from build123d import *

# Parameters (mm, degrees)
F0_R     = 1.5
F1_DEPTH = 1.5


# Not quite as in the source:
# - ends of sketch curves that miss each other by under 0.0002 mm in the source are joined


with BuildPart() as f1:
    # F0 (on Top) → F1 (new body)
    with BuildSketch(Plane.XY):
        with BuildLine():
            Line((-29.5, 6.644661), (-29.5, 0))
            Line((-29.5, 0), (-29.5, -6.644661))
            ThreePointArc((-29.5, -6.644661), (-30.4515057083, -11.4282035779), (-33.1611647352, -15.4834952648))
            Line((-33.1611647352, -15.4834952648), (-35.355339, -17.677669))
            Line((-35.355339, -17.677669), (-27.577165, -25.455844))
            ThreePointArc((-27.577165, -25.455844), (-25.4558450782, -25.4558435782), (-25.4558443282, -27.5771636718))
            Line((-25.4558443282, -27.5771636718), (-17.67767, -35.355339))
            ThreePointArc((-17.67767, -35.355339), (-3.536e-07, -28.033008), (17.6776695297, -35.3553384703))
            Line((17.6776695297, -35.3553384703), (25.455844, -27.577164))
            ThreePointArc((25.455844, -27.577164), (25.4558438282, -25.4558438282), (27.5771641718, -25.4558438282))
            Line((27.5771641718, -25.4558438282), (35.355339, -17.677669))
            Line((35.355339, -17.677669), (33.161165, -15.483495))
            ThreePointArc((33.161165, -15.483495), (30.4515057083, -11.4282035779), (29.5, -6.644661))
            Line((29.5, -6.644661), (29.5, 0))
            Line((29.5, 0), (29.5, 6.644661))
            ThreePointArc((29.5, 6.644661), (30.4515058436, 11.4282039046), (33.1611652352, 15.4834957648))
            Line((33.1611652352, 15.4834957648), (35.355339, 17.67767))
            Line((35.355339, 17.67767), (27.577164, 25.455844))
            ThreePointArc((27.577164, 25.455844), (25.4558435782, 25.4558450782), (25.4558438282, 27.5771651718))
            Line((25.4558438282, 27.5771651718), (17.677669, 35.355339))
            ThreePointArc((17.677669, 35.355339), (-3.536e-07, 28.033009), (-17.6776695297, 35.3553394703))
            Line((-17.6776695297, 35.3553394703), (-25.455844, 27.577165))
            ThreePointArc((-25.455844, 27.577165), (-25.4558448282, 25.4558448282), (-27.5771646718, 25.4558443282))
            Line((-27.5771646718, 25.4558443282), (-35.355339, 17.67767))
            Line((-35.355339, 17.67767), (-33.161165, 15.483496))
            ThreePointArc((-33.161165, 15.483496), (-30.4515058436, 11.4282039046), (-29.5, 6.644661))
        make_face()
        with Locations((-17.854446, -26.693281)):
            Circle(F0_R, mode=Mode.SUBTRACT)
        with Locations((-26.693281, -17.854446)):
            Circle(F0_R, mode=Mode.SUBTRACT)
        with Locations((-15.25, -15.25)):
            Circle(F0_R, mode=Mode.SUBTRACT)
        with Locations((17.854446, -26.693281)):
            Circle(F0_R, mode=Mode.SUBTRACT)
        with Locations((26.693281, -17.854446)):
            Circle(F0_R, mode=Mode.SUBTRACT)
        with Locations((15.25, -15.25)):
            Circle(F0_R, mode=Mode.SUBTRACT)
        with BuildLine():
            Line((11.5, -18), (-11.5, -18))
            ThreePointArc((-11.5, -18), (-12.2071067812, -17.7071067812), (-12.5, -17))
            Line((-12.5, -17), (-12.5, -15.25))
            ThreePointArc((-12.5, -15.25), (-13.3054563517, -13.3054563517), (-15.25, -12.5))
            Line((-15.25, -12.5), (-17, -12.5))
            ThreePointArc((-17, -12.5), (-17.7071067812, -12.2071067812), (-18, -11.5))
            Line((-18, -11.5), (-18, 11.5))
            ThreePointArc((-18, 11.5), (-17.7071067812, 12.2071067812), (-17, 12.5))
            Line((-17, 12.5), (-15.25, 12.5))
            ThreePointArc((-15.25, 12.5), (-13.3054563517, 13.3054563517), (-12.5, 15.25))
            Line((-12.5, 15.25), (-12.5, 17))
            ThreePointArc((-12.5, 17), (-12.2071067812, 17.7071067812), (-11.5, 18))
            Line((-11.5, 18), (11.5, 18))
            ThreePointArc((11.5, 18), (12.2071067812, 17.7071067812), (12.5, 17))
            Line((12.5, 17), (12.5, 15.25))
            ThreePointArc((12.5, 15.25), (13.3054563517, 13.3054563517), (15.25, 12.5))
            Line((15.25, 12.5), (17, 12.5))
            ThreePointArc((17, 12.5), (17.7071067812, 12.2071067812), (18, 11.5))
            Line((18, 11.5), (18, -11.5))
            ThreePointArc((18, -11.5), (17.7071067812, -12.2071067812), (17, -12.5))
            Line((17, -12.5), (15.25, -12.5))
            ThreePointArc((15.25, -12.5), (13.3054563517, -13.3054563517), (12.5, -15.25))
            Line((12.5, -15.25), (12.5, -17))
            ThreePointArc((12.5, -17), (12.2071067812, -17.7071067812), (11.5, -18))
        make_face(mode=Mode.SUBTRACT)
        with Locations((-15.25, 15.25)):
            Circle(F0_R, mode=Mode.SUBTRACT)
        with Locations((-26.693281, 17.854447)):
            Circle(F0_R, mode=Mode.SUBTRACT)
        with Locations((-17.854446, 26.693281)):
            Circle(F0_R, mode=Mode.SUBTRACT)
        with Locations((15.25, 15.25)):
            Circle(F0_R, mode=Mode.SUBTRACT)
        with Locations((26.693281, 17.854447)):
            Circle(F0_R, mode=Mode.SUBTRACT)
        with Locations((17.854446, 26.693281)):
            Circle(F0_R, mode=Mode.SUBTRACT)
    extrude(amount=F1_DEPTH)


solid = f1.part
Read the model definition and answer for the solid it produces. Units are mm, in the model's axes. A direction names the side the tool comes from. Give positions to 0.01 mm unless a question says otherwise; leave off trailing zeros. Write each loop counter-clockwise with the first axis right and the second up, starting at its lowest first coordinate (ties: lowest second). Pieces come first, ordered by that corner, then holes. Notation, with made-up numbers: (25.25, 45.25) -> (34.25, 45.25) arc R11 cw to (34.25, 57.25) -> close; hole circle Ø1 at (-3, 89). An arc over 180 degrees is marked (long way). Answer as a JSON object with one key per item and string values. Group by question number.
1) The mould has two halves that part along X. Classify faces 5 (the flat face through (-31.412, 21.621, 0.74)), 6 (the cylindrical face through (-0.275, -28.035, 0.74)), 7 (the cylindrical face through (13.75, -15.18, 0.74)), 8 (the flat face through (34.243, 16.565, 0.74)): +X half, -X half, draft (parallel to the pull), parting line (faces both ways), or undercut.
2) Find section A-A (y = -0.5). Write down the section's boundary in (x, z).
3) Each of these flat-tipped pins is pushed along its axis until it touches: P1, Ø2.5, axis at x = -26.69, y = 17.85, coming from the +Z side; P2, Ø0.8, axis at y = 1, z = 1, coming from the -X side; P3, Ø0.8, axis at y = 1.5, z = 1, coming from the +X side. Where does it stop, or does it pass through?
4) Find section D-D (y = 23). Write down the section's boundary in (x, z).
5) Find section C-C (z = 0.35). Count the separate pieces of the cut face and the enclosed holes in it, and give its area (3 significant figures).
6) A tool of negligible diameter and unlimited length cuts with its end or side. For faces 1 (the cylindrical face through (0.275, 28.035, 0.74)), 2 (the cylindrical face through (13.28, 13.33, 0.74)), 3 (the flat face through (-34.274, 16.596, 0.74)), 4 (the cylindrical face through (30.478, -11.492, 0.74)), from which of +Z, -Z, +X, -X, +Y, -Y can it reach the whole face along a straight path? Write none if from no direction.
7) Find section B-B (x = -2). Write down the section's boundary in (y, z), and give its area (3 significant figures).
8) Consider L1, parallel to Y at x = 26.5, z = 0.5; L2, parallel to X at y = 15.5, z = 1.4; L3, parallel to X at y = 28, z = 0.4. Determine where each line is inside the solid, lowest interval first. Write a range as from..to.
Values follow:
{
 "1": {"face 5": "-X half", "face 6": "undercut", "face 7": "undercut", "face 8": "+X half"},
 "2": {"outline": "(-29.5, 0) -> (-18, 0) -> (-18, 1.5) -> (-29.5, 1.5) -> close; (18, 0) -> (29.5, 0) -> (29.5, 1.5) -> (18, 1.5) -> close"},
 "3": {"P1": "passes through", "P2": "stops at x = -29.5", "P3": "stops at x = 29.5"},
 "4": {"outline": "(-30.03, 0) -> (30.03, 0) -> (30.03, 1.5) -> (-30.03, 1.5) -> close"},
 "5": {"separate pieces": "1", "enclosed holes": "13", "area": "2,410 mm2"},
 "6": {"face 1": "+Z, -Z, +Y", "face 2": "+Z, -Z", "face 3": "+Z, -Z, -X", "face 4": "+Z, -Z, +X"},
 "7": {"outline": "(-28.11, 0) -> (-18, 0) -> (-18, 1.5) -> (-28.11, 1.5) -> close; (18, 0) -> (28.11, 0) -> (28.11, 1.5) -> (18, 1.5) -> close", "area": "30.3 mm2"},
 "8": {"L1": "y = -25.02..-19.34, -16.37..16.37, 19.34..25.02", "L2": "x = -33.18..-16.73, -13.77..-12.5, 12.5..13.77, 16.73..33.18", "L3": "x = -25.03..-18.59, -17.12..17.12, 18.59..25.03"}
}
